Check sheet for the modelled part. Datum: model origin and axes. Units: mm. A direction names the side the tool comes from. Coordinates: 2 decimals unless noted, no trailing zeros. Write each loop counter-clockwise with the first axis right and the second up, starting at its lowest first coordinate (ties: lowest second). Pieces come first, ordered by that corner, then holes. Notation, with made-up numbers: M -18,80 L 32,80 A16 cw 32,102 Z; hole C -10.5,57.25 d8. An arc over 180 degrees is marked long. Answer as CSV lines item,"result". Start each with the question number.
Q1. Sectioned sample at C-C, the plane y = 377. Record the cut outline in (x, z).
Q2. Access from +Z, -Z, +X, -X, +Y, -Y to the whole of each face (thin tool, end or side, straight path). Record for faces 1 (the flat face through (-50.304, 202, 162)), 2 (the flat face through (30, 202, 117.802)), 3 (the flat face through (-79.804, -5, -68)), 4 (the flat face through (-2, 202, 179.802)).
Q3. Sectioned sample at B-B, the plane z = -72. Record the cut outline in (x, y).
Q4. Thickness scan on line 1 along Z through (x, y) = (-36, 372.5); line 2 along X through (y, z) = (207, 164); line 3 along Y through (x, z) = (-44.5, 150.5). Record the ranges inside material, lowest first. Write a range as from..to.
Q5. Mould release check, pull along X, two halves, no side actions. Record for faces 5 (the flat face through (-35, 202, 117.802)), 6 (the flat face through (-34, 202, 120.802)), 7 (the flat face through (41.696, 202, 161)), 8 (the flat face through (-99.804, -5, 32)): pulls with the +X half, pulls with the -X half, needs draft (parallel to the pull), parting line crosses it, or undercut.
Q6. Sectioned sample at D-D, the plane x = -11.5. Record the cut outline in (y, z), then the cut area to 3 significant figures.
Q7. Depth check by flat-ended pin: pin 1 Ø23 at (y, z) = (205, 150.3) entering from -X; pin 2 Ø11.5 at (x, z) = (84.2, -107.2) entering from -Y; pin 3 Ø6 at (x, z) = (16, 140) entering from +Y; pin 4 Ø9 at (x, z) = (-89.8, 167.8) entering from +Y. Enter the tip coordinate at first touch or a pass-through.
Q8. Sectioned sample at A-A, the plane y = 205. Record the cut outline in (x, z).
from build123d import *

# Parameters (mm, degrees)
F1_DEPTH = 10
F3_DEPTH = 410
F4_R     = 5
F5_R     = 5
F6_R     = 5
F7_DEPTH = 10.001
F8_R     = 10
F9_DEPTH = 144.501


with BuildPart() as f1:
    # F0 (on Front) → F1 (new body)
    with BuildSketch(Plane.XZ):
        with BuildLine():
            Line((-79.8040040345, -122.1982348855), (-79.8040040345, -17.0901585641))
            ThreePointArc((-79.8040040345, -17.0901585641), (-2.8040040345, 59.9098414359), (74.1959959655, -17.0901585641))
            Line((74.1959959655, -17.0901585641), (74.1959959655, -122.1982348855))
            Line((74.1959959655, -122.1982348855), (94.1959959655, -122.1982348855))
            Line((94.1959959655, -122.1982348855), (94.1959959655, 182.8017651145))
            Line((94.1959959655, 182.8017651145), (-99.8040040345, 182.8017651145))
            Line((-99.8040040345, 182.8017651145), (-99.8040040345, -122.1982348855))
            Line((-99.8040040345, -122.1982348855), (-79.8040040345, -122.1982348855))
        make_face()
    extrude(amount=F1_DEPTH)

    # F2 (on face) → F3 (join)
    with BuildSketch(Plane(origin=(0, 0, 0), x_dir=(-1, 0, 0), z_dir=(0, 1, 0))):
        Polygon((50.3040040345, 117.8017651145), (50.3040040345, 182.8017651145), (-44.6959959655, 182.8017651145), (-44.6959959655, 117.8017651145), (-19.6959959655, 117.8017651145), (-19.6959959655, 120.8017651145), (-41.6959959655, 120.8017651145), (-41.6959959655, 179.8017651145), (47.3040040345, 179.8017651145), (47.3040040345, 120.8017651145), (25.3040040345, 120.8017651145), (25.3040040345, 117.8017651145), align=None)
    extrude(amount=F3_DEPTH)

    # F4
    f4_edges = [f1.edges().sort_by_distance(p)[0] for p in [
        (44.695996, 205, 182.801765),
        (-50.304004, 205, 182.801765),
        (-50.304004, 205, 117.801765),
        (44.695996, 205, 117.801765),
        (-47.304004, 205, 179.801765),
        (-47.304004, 205, 120.801765),
        (41.695996, 205, 120.801765),
        (41.695996, 205, 179.801765),
    ]]
    fillet(f4_edges, radius=F4_R)

    # F5
    f5_edges = [f1.edges().sort_by_distance(p)[0] for p in [
        (-99.804004, -5, -122.198235),
        (-99.804004, -5, 182.801765),
        (94.195996, -5, 182.801765),
        (94.195996, -5, -122.198235),
        (74.195996, -5, -122.198235),
        (-79.804004, -5, -122.198235),
    ]]
    fillet(f5_edges, radius=F5_R)

    # F6 (on face) → F7 (cut, through all)
    with BuildSketch(Plane(origin=(0, 0, 0), x_dir=(-1, 0, 0), z_dir=(0, 1, 0))):
        with Locations((-84.1959959655, 167.8017651145)):
            Circle(F6_R)
        with Locations((-84.1959959655, 30.3017651145)):
            Circle(F6_R)
        with Locations((-84.1959959655, -107.1982348855)):
            Circle(F6_R)
        with Locations((89.8040040345, 167.8017651145)):
            Circle(F6_R)
        with Locations((89.8040040345, 30.3017651145)):
            Circle(F6_R)
        with Locations((89.8040040345, -107.1982348855)):
            Circle(F6_R)
    extrude(amount=-F7_DEPTH, mode=Mode.SUBTRACT)

    # F8 (on face) → F9 (cut, through all)
    with BuildSketch(Plane.YZ.offset(44.6959959655)):
        with Locations((205, 150.3017651145)):
            Circle(F8_R)
    extrude(amount=-F9_DEPTH, mode=Mode.SUBTRACT)


solid = f1.part
Output:
1,outline,"M -50.3,122.8 A5 ccw -45.3,117.8 L -25.3,117.8 L -25.3,120.8 L -42.3,120.8 A5 cw -47.3,125.8 L -47.3,174.8 A5 cw -42.3,179.8 L 36.7,179.8 A5 cw 41.7,174.8 L 41.7,125.8 A5 cw 36.7,120.8 L 19.7,120.8 L 19.7,117.8 L 39.7,117.8 A5 ccw 44.7,122.8 L 44.7,177.8 A5 ccw 39.7,182.8 L -45.3,182.8 A5 ccw -50.3,177.8 Z"
2,face 1,"+Z, -Z, -X, +Y"
2,face 2,"-Z, +X, -X, +Y"
2,face 3,"-Z, +Y, -Y"
2,face 4,"+Y"
3,outline,"M -99.8,-10 L -79.8,-10 L -79.8,0 L -99.8,0 Z; M 74.2,-10 L 94.2,-10 L 94.2,0 L 74.2,0 Z"
4,line 1,"z = 117.8..120.8, 179.8..182.8"
4,line 2,"x = -50.3..-47.3, 41.7..44.7"
4,line 3,"y = -10..0"
5,face 5,"needs draft"
5,face 6,"undercut"
5,face 7,"undercut"
5,face 8,"pulls with the -X half"
6,outline,"M -10,59.42 L 0,59.42 L 0,179.8 L 410,179.8 L 410,182.8 L -10,182.8 Z"
6,area,"2,460 mm^2"
7,pin 1,"stops at x = -50.3"
7,pin 2,"stops at y = -10"
7,pin 3,"stops at y = 0"
7,pin 4,"passes through"
8,outline,"M -50.3,122.8 A5 ccw -45.3,117.8 L -25.3,117.8 L -25.3,120.8 L -42.3,120.8 A5 cw -47.3,125.8 L -47.3,140.3 L -50.3,140.3 Z; M -50.3,160.3 L -47.3,160.3 L -47.3,174.8 A5 cw -42.3,179.8 L 36.7,179.8 A5 cw 41.7,174.8 L 41.7,160.3 L 44.7,160.3 L 44.7,177.8 A5 ccw 39.7,182.8 L -45.3,182.8 A5 ccw -50.3,177.8 Z; M 19.7,117.8 L 39.7,117.8 A5 ccw 44.7,122.8 L 44.7,140.3 L 41.7,140.3 L 41.7,125.8 A5 cw 36.7,120.8 L 19.7,120.8 Z"
